Source: CAD feature listing. Evaluate the final solid. Frame: model axes, mm. Face numbers are marked on the shaded views. A direction names the side the tool comes from. Give positions to 0.01 mm unless a question says otherwise; leave off trailing zeros. Loops run counter-clockwise (first coordinate to the right, second up) from the corner with the lowest first, then second, coordinate; pieces in that order, holes last.
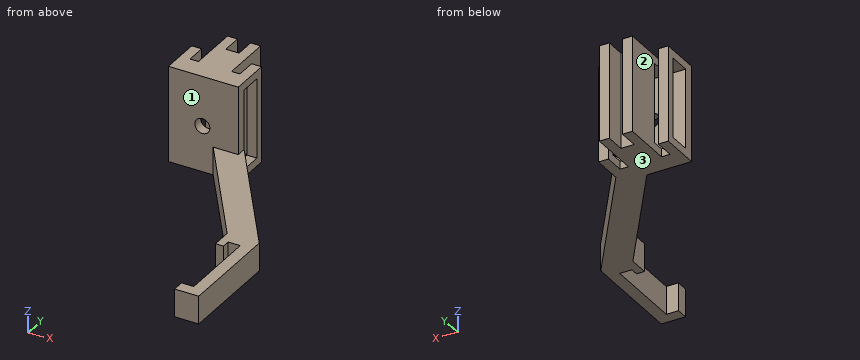
Autodesk Inventor part; units mm, degrees
ref_plane "YZ Plane" through (0, 0, 0) normal (1, 0, 0) x (0, 1, 0)
ref_plane "XZ Plane" through (0, 0, 0) normal (0, 1, 0) x (-1, 0, 0)
ref_plane "XY Plane" through (0, 0, 0) normal (0, 0, 1) x (1, 0, 0)
sketch "Náčrt1" plane through (0, 0, 0) normal (0, 0, 1) x (1, 0, 0)
  line L0 (21, 22) -> (21, -30)
  line L1 (21, -30) -> (8.9, -30)
  line L2 (8.9, -30) -> (8.9, -24)
  line L3 (8.9, -24) -> (15, -24)
  line L4 (15, -24) -> (15, 16)
  line L5 (15, 16) -> (8.9, 16)
  line L6 (8.9, 16) -> (8.9, 12)
  line L7 (8.9, 12) -> (4.9, 12)
  line L8 (4.9, 12) -> (4.9, 22)
  line L9 (4.9, 22) -> (-37.1125, 82)
  line L10 (-24.5135, 87) -> (21, 22)
  line L11 (-37.1125, 82) -> (-59.5135, 82)
  line L12 (-59.5135, 82) -> (-59.5135, 87)
  line L13 (-59.5135, 87) -> (-24.5135, 87)
  point P0 (0, 0)
  dimension "d10" = 40
  dimension "d14" = 6.1
  dimension "d15" = 4
  dimension "d16" = 4
  dimension "d28" = 6
  dimension "d29" = 12.1
  dimension "d30" = 6
  dimension "d31" = 6.1
  dimension "d32" = 145
  dimension "d33" = 15
  dimension "d34" = 145
  dimension "d35" = 52
  dimension "d36" = 10
  dimension "d37" = 30
  dimension "d40" = 60
  dimension "d41" = 65
  dimension "d43" = 35
  dimension "d44" = 5
extrude "Vysunutí1" add sketch "Náčrt1" along normal blind 6 and the other way blind 4
sketch "Náčrt2" plane through (0, 0, 6) normal (0, 0, 1) x (1, 0, 0)
  line L0 (-59.5135, 82) -> (-37.1125, 82)
  line L1 (-24.5135, 87) -> (-59.5135, 87)
  line L2 (-59.5135, 82) -> (-24.5135, 82)
  line L3 (-24.5135, 82) -> (-24.5135, 87)
  line L4 (-24.5135, 87) -> (-59.5135, 87)
  line L5 (-59.5135, 87) -> (-59.5135, 82)
  point P0 (0, 0)
extrude "Vysunutí2" add sketch "Náčrt2" along normal blind 30
sketch "Náčrt3" plane through (-59.5135, 87, -4) normal (0, 1, 0) x (1, 0, 0)
  circle A0 centre (17, -19) radius 3.75
  line L0 (0, 0) -> (35, 0)
  line L1 (35, -10) -> (35, -40)
  point P0 (59.5135, -4)
  dimension "d49" = 7.5
  dimension "d50" = 19
  dimension "d51" = 18
extrude "Vysunutí3" cut sketch "Náčrt3" against normal blind 30
sketch "Náčrt4" plane through (-59.5135, 82, -4) normal (0, -1, 0) x (1, 0, 0)
  line L0 (0, 40) -> (35, 40)
  line L1 (35, 40) -> (0, 40)
  line L2 (0, 40) -> (0, 44)
  line L3 (0, 44) -> (35, 44)
  line L4 (35, 44) -> (35, 40)
  line L5 (0, 0) -> (35, 0)
  line L6 (35, 0) -> (35, -4)
  line L7 (35, -4) -> (0, -4)
  line L8 (0, -4) -> (0, 0)
  line L9 (22.401, 0) -> (0, 0)
  point P0 (59.5135, 4)
  dimension "d54" = 4
  dimension "d55" = 4
  dimension "d57" = 35
  dimension "d58" = 35
extrude "Vysunutí4" add sketch "Náčrt4" against normal blind 16
sketch "Náčrt5" plane through (-59.5135, 82, 40) normal (0, 0, 1) x (1, 0, 0)
  line L0 (0, 16) -> (35, 16)
  line L1 (0, 16) -> (35, 16)
  line L2 (35, 16) -> (35, 20)
  line L3 (35, 20) -> (0, 20)
  line L4 (0, 20) -> (0, 16)
  point P0 (59.5135, -82)
  dimension "d61" = 35
  dimension "d62" = 4
extrude "Vysunutí5" add sketch "Náčrt5" against normal blind 48
sketch "Náčrt6" plane through (-59.5135, 82, 40) normal (0, 0, 1) x (1, 0, 0)
  line L0 (5, 20) -> (9.2, 20)
  line L1 (9.2, 20) -> (9.2, 10)
  line L2 (9.2, 10) -> (5, 10)
  line L3 (5, 10) -> (5, 20)
  line L4 (25.8, 20) -> (30, 20)
  line L5 (30, 20) -> (30, 10)
  line L6 (30, 10) -> (25.8, 10)
  line L7 (25.8, 10) -> (25.8, 20)
  line L8 (35, 20) -> (0, 20)
  line L9 (0, 0) -> (0, 20)
  line L10 (35, 0) -> (35, 20)
  point P0 (59.5135, -82)
  dimension "d65" = 5
  dimension "d66" = 4.2
  dimension "d67" = 5
  dimension "d68" = 4.2
  dimension "d69" = 10
  dimension "d70" = 10
extrude "Vysunutí6" cut sketch "Náčrt6" against normal blind 50
sketch "Náčrt8" plane through (-50.3135, 102, 40) normal (0, 1, 0) x (1, 0, 0)
  line L0 (0, 48) -> (0, 0)
  line L1 (16.6, 0) -> (0, 0)
  line L2 (0, 48) -> (16.6, 48)
  line L3 (16.6, 48) -> (16.6, 0)
  line L4 (16.6, 0) -> (0, 0)
  line L5 (0, 0) -> (0, 48)
  point P0 (50.3135, 40)
extrude "Vysunutí7" add sketch "Náčrt8" along normal blind 5
sketch "Náčrt9" plane through (-50.3135, 107, 40) normal (0, 1, 0) x (1, 0, 0)
  line L0 (0, 48) -> (0, 0)
  line L1 (25.8, 0) -> (-9.2, 0)
  line L2 (0, 48) -> (5, 48)
  line L3 (5, 48) -> (5, 0)
  line L4 (5, 0) -> (0, 0)
  line L5 (0, 0) -> (0, 48)
  line L6 (16.6, 48) -> (11.6, 48)
  line L7 (11.6, 48) -> (11.6, 0)
  line L8 (11.6, 0) -> (16.6, 0)
  line L9 (16.6, 0) -> (16.6, 48)
  point P0 (50.3135, 40)
  point P1 (16.6, 0)
  dimension "d75" = 5
  dimension "d76" = 5
extrude "Vysunutí8" add sketch "Náčrt9" along normal blind 10
sketch "Náčrt11" plane through (0, 0, -4) normal (0, 0, -1) x (-1, 0, 0)
  line L0 (37.1125, 82) -> (-4.9, 22)
  line L1 (37.1125, 82) -> (-4.9, 22)
  line L2 (-4.9, 22) -> (-4.9, 12)
  line L3 (-4.9, 22) -> (-4.9, 12)
  line L4 (-4.9, 12) -> (-8.9, 12)
  line L5 (-4.9, 12) -> (-8.9, 12)
  line L6 (-8.9, 12) -> (-8.9, 16)
  line L7 (-8.9, 12) -> (-8.9, 16)
  line L8 (-8.9, 16) -> (-15, 16)
  line L9 (-8.9, 16) -> (-15, 16)
  line L10 (-15, 16) -> (-15, -24)
  line L11 (-15, 16) -> (-15, -24)
  line L12 (-15, -24) -> (-8.9, -24)
  line L13 (-15, -24) -> (-8.9, -24)
  line L14 (-8.9, -24) -> (-8.9, -30)
  line L15 (-8.9, -24) -> (-8.9, -30)
  line L16 (-8.9, -30) -> (-21, -30)
  line L17 (-8.9, -30) -> (-21, -30)
  line L18 (-21, -30) -> (-21, 22)
  line L19 (-21, -30) -> (-21, 22)
  line L20 (24.5135, 87) -> (59.5135, 87)
  line L21 (-21, 22) -> (24.5135, 87)
  line L22 (24.5135, 82) -> (24.5135, 102)
  line L23 (24.5135, 87) -> (24.5135, 82)
  line L24 (24.5135, 82) -> (37.1125, 82)
  line L25 (24.5135, 82) -> (59.5135, 82)
  point P0 (0, 0)
extrude "Vysunutí9" add sketch "Náčrt11" along normal blind 4
properties part number "DrzakKamera"
1) Cut plane C-C (y = 85). Return loops of the section in (x, z), and give its area (3 significant figures).
Checks:
outline: (-59.51, -8) - (-23.11, -8) - (-23.11, 6) - (-24.51, 6) - (-24.51, 40) - (-59.51, 40) - close; hole circle Ø7.5 at (-42.51, 15)
area: 1,660 mm2
2) Cut plane D-D (x = -10). Return loops of the section in (y, z).
Checks:
outline: (43.28, -8) - (66.27, -8) - (66.27, 6) - (43.28, 6) - close
3) Reachability of the marked faces 1, 2 and 3 from +Z, -Z, +X, -X, +Y, -Y: full face, straight path, thin tool, end or side. Return the list, or none.
Checks:
face 1: +Z, -X, -Y
face 2: +Z, -Z, +Y
face 3: -Z, +X, -X, +Y, -Y
4) Ray query, probe 1 along X at (y, z) = (84, 15); probe 2 along Y at (x, z) = (13, -3); probe 3 along Y at (x, z) = (-48, 16). Return the intervals inside material, ascending.
Checks:
probe 1: x = -59.51 to -46.26, -38.76 to -24.51
probe 2: y = -30 to -24, 16 to 33.43
probe 3: y = 82 to 87, 98 to 117
5) Contact query for flat-ended pins moving along their axis: P1, Ø3, axis at y = 110, z = 14.5, coming from the +X side; P2, Ø1.2, axis at x = -31, z = -6, coming from the +Y side; P3, Ø5.5, axis at x = -57, z = 9, coming from the -Y side. Output: stop coordinate, or through.
Checks:
P1: stops at x = -33.71
P2: stops at y = 92
P3: stops at y = 82
6) Cut plane A-A (z = 8). Return loops of the section in (x, y), and give its area (3 significant figures).
Checks:
outline: (-59.51, 82) - (-24.51, 82) - (-24.51, 87) - (-59.51, 87) - close; (-59.51, 98) - (-54.51, 98) - (-54.51, 102) - (-59.51, 102) - close; (-50.31, 98) - (-33.71, 98) - (-33.71, 117) - (-38.71, 117) - (-38.71, 107) - (-45.31, 107) - (-45.31, 117) - (-50.31, 117) - close; (-29.51, 98) - (-24.51, 98) - (-24.51, 102) - (-29.51, 102) - close
area: 464 mm2
7) Cut plane B-B (z = 15). Return loops of the section in (x, y), and give its area (3 significant figures).
Checks:
outline: (-59.51, 82) - (-46.26, 82) - (-46.26, 87) - (-59.51, 87) - close; (-59.51, 98) - (-54.51, 98) - (-54.51, 102) - (-59.51, 102) - close; (-50.31, 98) - (-33.71, 98) - (-33.71, 117) - (-38.71, 117) - (-38.71, 107) - (-45.31, 107) - (-45.31, 117) - (-50.31, 117) - close; (-38.76, 82) - (-24.51, 82) - (-24.51, 87) - (-38.76, 87) - close; (-29.51, 98) - (-24.51, 98) - (-24.51, 102) - (-29.51, 102) - close
area: 427 mm2
